from build123d import *

# Parameters (mm, degrees)
F1_DEPTH = 63.5
F2_DEPTH = 25.4
F3_DEPTH = 7.9375
F5_DEPTH = 12.7
F6_R     = 5.08


with BuildPart() as f1:
    # F0 (on Front) → F1 (new body, symmetric)
    with BuildSketch(Plane.XZ):
        Polygon((-41.275, -9.525), (41.275, -9.525), (41.275, 9.525), (22.225, 9.525), (-41.275, 9.525), align=None)
    extrude(amount=F1_DEPTH, both=True)

    # F0 (on Front) → F2 (join, symmetric)
    with BuildSketch(Plane.XZ):
        with BuildLine():
            Line((22.225, 9.525), (41.275, 9.525))
            Line((41.275, 9.525), (41.275, 27.0002))
            ThreePointArc((41.275, 27.0002), (45.9246798487, 38.2255201513), (57.15, 42.8752))
            Line((57.15, 42.8752), (60.325, 42.8752))
            Line((60.325, 42.8752), (60.325, 61.9252))
            Line((60.325, 61.9252), (57.15, 61.9252))
            add(Edge.make_bspline(
                [(51.1085881946, 61.398702415), (53.7307154629, 61.6641570912), (55.7925510504, 61.8177418079), (57.15, 61.9252)],
                knots=[0.7544555653, 0.7544555653, 0.7544555653, 0.7544555653, 0.8556201459, 0.8556201459, 0.8556201459, 0.8556201459], degree=3))
            ThreePointArc((51.1085881946, 61.398702415), (30.4034868412, 49.4585984034), (22.225, 27.0002))
            Line((22.225, 27.0002), (22.225, 9.525))
        make_face()
        Polygon((60.325, 61.9252), (60.325, 42.8752), (85.729400427, 42.8752), (85.7469553221, 61.9252), align=None)
    extrude(amount=F2_DEPTH, both=True)

    # F0 (on Front) → F3 (join, symmetric)
    with BuildSketch(Plane.XZ):
        with BuildLine():
            add(Edge.make_bspline(
                [(-41.275, 9.525), (-19.1634568795, 51.2174255763), (31.5535374202, 59.4190198373), (51.1085881946, 61.398702415)],
                knots=[0, 0, 0, 0, 0.7544555653, 0.7544555653, 0.7544555653, 0.7544555653], degree=3))
            Line((-41.275, 9.525), (22.225, 9.525))
            Line((22.225, 9.525), (22.225, 27.0002))
            ThreePointArc((22.225, 27.0002), (30.4034868412, 49.4585984034), (51.1085881946, 61.398702415))
        make_face()
    extrude(amount=F3_DEPTH, both=True)

    # F0 (on Front) → F4 (revolve)
    with BuildSketch(Plane.XZ):
        Polygon((85.7469553221, 61.9252), (85.729400427, 42.8752), (85.725, 38.1), (111.125, 38.1), (111.125, 66.675), (85.7513323426, 66.675), align=None)
    revolve(axis=Axis((85.7381661713, 0, 52.3875), (0.0009215164, 0, 0.9999995754)))

    # F0 (on Front) → F5 (join, symmetric)
    with BuildSketch(Plane.XZ):
        with BuildLine():
            Line((22.225, 9.525), (41.275, 9.525))
            Line((41.275, 9.525), (41.275, 27.0002))
            ThreePointArc((41.275, 27.0002), (45.9246798487, 38.2255201513), (57.15, 42.8752))
            Line((57.15, 42.8752), (60.325, 42.8752))
            Line((60.325, 42.8752), (60.325, 61.9252))
            Line((60.325, 61.9252), (57.15, 61.9252))
            add(Edge.make_bspline(
                [(51.1085881946, 61.398702415), (53.7307154629, 61.6641570912), (55.7925510504, 61.8177418079), (57.15, 61.9252)],
                knots=[0.7544555653, 0.7544555653, 0.7544555653, 0.7544555653, 0.8556201459, 0.8556201459, 0.8556201459, 0.8556201459], degree=3))
            ThreePointArc((51.1085881946, 61.398702415), (30.4034868412, 49.4585984034), (22.225, 27.0002))
            Line((22.225, 27.0002), (22.225, 9.525))
        make_face()
    extrude(amount=F5_DEPTH, both=True)

    # F6
    f6_edges = [f1.edges().sort_by_distance(p)[0] for p in [
        (41.275, -63.5, 0),
        (-41.275, -63.5, 0),
        (41.275, 63.5, 0),
        (-41.275, 63.5, 0),
    ]]
    fillet(f6_edges, radius=F6_R)


solid = f1.part
Read the model definition and answer for the solid it produces. Units are mm, in the model's axes. A direction names the side the tool comes from. Give positions to 0.01 mm unless a question says otherwise; leave off trailing zeros. Write each loop counter-clockwise with the first axis right and the second up, starting at its lowest first coordinate (ties: lowest second). Pieces come first, ordered by that corner, then holes. Notation, with made-up numbers: (24, -19.5) - (65, -19.5) arc R7 ccw to (65, -9.5) - close; hole circle Ø4 at (0, -16). An arc over 180 degrees is marked (long way). Answer in a Markdown table with one row per item. Add a question column.
Item 1: Section B-B, the plane y = 32 is taken. Write down the section's boundary in (x, z) (3 decimals), and give its area (3 significant figures).
Item 2: A tool of negligible diameter and unlimited length cuts with its end or side. For faces 1 (the face through (60, 2, 42.875)), 2 (the face through (45.8, -0.4, 38.1)), 3 (the face through (46, -25.4, 42)), 4 (the face through (-5, -7.938, 30)), 5 (the face through (60, 0, 61.925)), from which of +Z, -Z, +X, -X, +Y, -Y can it reach the whole face along a straight path? Write none if from no direction.
Item 3: Find the intervals of material crossed by L1, parallel to Z at x = -16.5, y = -8 (3 decimals); L2, parallel to Y at x = 41, z = 31; L3, parallel to Y at x = 28, z = 50.5, in increasing order.
Item 4: Section A-A, the plane z = -4 is taken. Write down the section's boundary in (x, y) (3 decimals).
Item 5: Flat-ended cylindrical pins translate along their axes: P1, Ø1.5, axis at y = 3.5, z = 2, coming from the +X side (3 decimals); P2, Ø16.5, axis at x = 1, y = -36.5, coming from the +Z side (3 decimals); P3, Ø10, axis at y = 1, z = 51.5, coming from the -X side. Find the tip coordinate at first contact, or state that the pin passes through.
Recorded:
| question | item | result |
|---|---|---|
| 1 | outline | (-41.275, -9.525) - (41.275, -9.525) - (41.275, 9.525) - (-41.275, 9.525) - close |
| 1 | area | 1,570 mm2 |
| 2 | face 1 | -Z |
| 2 | face 2 | -Z, +Y, -Y |
| 2 | face 3 | +Z, +X, -X, -Y |
| 2 | face 4 | +Z, -X, -Y |
| 2 | face 5 | +Z, -X |
| 3 | L1 | z = -9.525 to 9.525 |
| 3 | L2 | y = -25.4 to 25.4 |
| 3 | L3 | y = -7.94 to 7.94 |
| 4 | outline | (-41.275, -58.42) arc R5.08 ccw to (-36.195, -63.5) - (36.195, -63.5) arc R5.08 ccw to (41.275, -58.42) - (41.275, 58.42) arc R5.08 ccw to (36.195, 63.5) - (-36.195, 63.5) arc R5.08 ccw to (-41.275, 58.42) - close |
| 5 | P1 | stops at x = 41.275 |
| 5 | P2 | stops at z = 9.525 |
| 5 | P3 | stops at x = -2.42 |
